Autodesk Inventor part; units mm, degrees
ref_plane "YZ Plane" through (0, 0, 0) normal (1, 0, 0) x (0, 1, 0)
ref_plane "XZ Plane" through (0, 0, 0) normal (0, 1, 0) x (-1, 0, 0)
ref_plane "XY Plane" through (0, 0, 0) normal (0, 0, 1) x (1, 0, 0)
sketch "Sketch1" plane through (0, 0, 0) normal (0, 1, 0) x (-1, 0, 0)
  line L0 (0, 0) -> (25, 0)
  line L1 (25, 0) -> (25, -25)
  line L2 (25, -25) -> (0, -25)
  line L3 (0, -25) -> (0, 0)
  dimension "d0" = 25
  dimension "d1" = 25
extrude "Extrusion1" add sketch "Sketch1" along normal blind 2
fillet "Fillet1" radius 2 4 edges at (0, 1, 0) (0, 1, -25) (-25, 1, 0) (-25, 1, -25)
sketch "Sketch2" plane through (0, 2, 0) normal (0, 1, 0) x (1, 0, 0)
  line L0 (-19, 25) -> (-19, 0)
  line L1 (-25, 23) -> (-25, 2)
  line L2 (-14, 25) -> (-14, 0)
  line L3 (-19, 25) -> (-14, 25)
  line L4 (-2, 25) -> (-23, 25)
  line L5 (-19, 0) -> (-14, 0)
  line L6 (-23, 0) -> (-2, 0)
  point P0 (0, 0)
  dimension "d5" = 6
  dimension "d6" = 5
extrude "Extrusion2" add sketch "Sketch2" along normal blind 3.9
sketch "Sketch4" plane through (0, 2, 0) normal (0, 1, 0) x (1, 0, 0)
  line L0 (-2, 25) -> (-14, 25)
  line L1 (0, 2) -> (0, 23)
  circle A0 centre (-7, 7) radius 2.5
  line L2 (-14, 0) -> (-2, 0)
  point P0 (0, 0)
  dimension "d11" = 5
  dimension "d14" = 7
  dimension "d15" = 7
extrude "Extrusion3" add sketch "Sketch4" along normal blind 10
properties part number "tapa_canyon_cambio"
The model under review builds one solid part; all positions refer to its coordinate system, in mm. A direction names the side the tool comes from. Round coordinates to 2 decimals unless told otherwise and drop trailing zeros. Order: outer loops, then holes, each group sorted by start corner. A loop starts at its lowest first (then second) coordinate and runs counter-clockwise, first axis right, second up. Notation, with made-up numbers: M -17,46 L -9,46 A28 cw -9,80 Z; hole C -15,-16.75 d4. An arc over 180 degrees is marked long. Use a Markdown table: item, result.
1) Consider section B-B (x = -7). Write out the cut boundary in (y, z).
Report:
| item | result |
|---|---|
| outline | M 0,-25 L 2,-25 L 2,-9.5 L 12,-9.5 L 12,-4.5 L 2,-4.5 L 2,0 L 0,0 Z |
2) Consider section C-C (y = 4.5). Write out the cut boundary in (x, z), then the cut area to 3 significant figures.
Report:
| item | result |
|---|---|
| outline | M -19,-25 L -14,-25 L -14,0 L -19,0 Z; C -7,-7 d5 |
| area | 145 mm^2 |
3) Wall thickness on line 1 along Y through (x, z) = (-19.75, -1.5); line 2 along Y through (x, z) = (-18, -11); line 3 along X through (y, z) = (5, -22): over which ranges is each line inside the solid? List them lowest first. Write a range as [from, to].
Report:
| item | result |
|---|---|
| line 1 | [0, 2] |
| line 2 | [0, 5.9] |
| line 3 | [-19, -14] |
4) Consider section D-D (z = -7). Write out the cut boundary in (x, y), then the cut area to 4 significant figures.
Report:
| item | result |
|---|---|
| outline | M -25,0 L 0,0 L 0,2 L -4.5,2 L -4.5,12 L -9.5,12 L -9.5,2 L -14,2 L -14,5.9 L -19,5.9 L -19,2 L -25,2 Z |
| area | 119.5 mm^2 |
5) Consider section A-A (z = -17.75). Write out the cut boundary in (x, y).
Report:
| item | result |
|---|---|
| outline | M -25,0 L 0,0 L 0,2 L -14,2 L -14,5.9 L -19,5.9 L -19,2 L -25,2 Z |
6) Tool access review of faces 1 (the face through (-12.4, 1.6, 0)), 2 (the face through (-22, 2, -12)): name each direction out of +Z, -Z, +X, -X, +Y, -Y from which nothing blocks a thin tool from reaching the whole face with its end or side.
Report:
| item | result |
|---|---|
| face 1 | +Z, +X, -X, +Y, -Y |
| face 2 | +Z, -Z, -X, +Y |
7) Insertion check: pin 1 (3 mm diameter, centred on y = 4, z = -15.5, fed in from -X); pin 2 (4 mm diameter, centred on x = -5.5, z = -16.5, fed in from +Y); pin 3 (5 mm diameter, centred on x = -15, y = 9, fed in from +Z); pin 4 (4 mm diameter, centred on x = -16, z = -10.5, fed in from +Y). Each pin has a flat end and moves straight along its axis. Give the tip position at first contact, or say it passes through.
Report:
| item | result |
|---|---|
| pin 1 | x = -19 |
| pin 2 | y = 2 |
| pin 3 | through |
| pin 4 | y = 5.9 |
8) Draft analysis for pull direction X (two halves, no side actions). For faces 3 (the face through (-19, 4, -13)), 4 (the face through (-5.85, 6.93, -9.22)), 5 (the face through (-17, 5.9, -13)), 6 (the face through (0, 1, -13)), state which applies: released by +X, released by -X, zero draft, split by the parting line, or undercut.
Report:
| item | result |
|---|---|
| face 3 | released by -X |
| face 4 | undercut |
| face 5 | zero draft |
| face 6 | released by +X |
